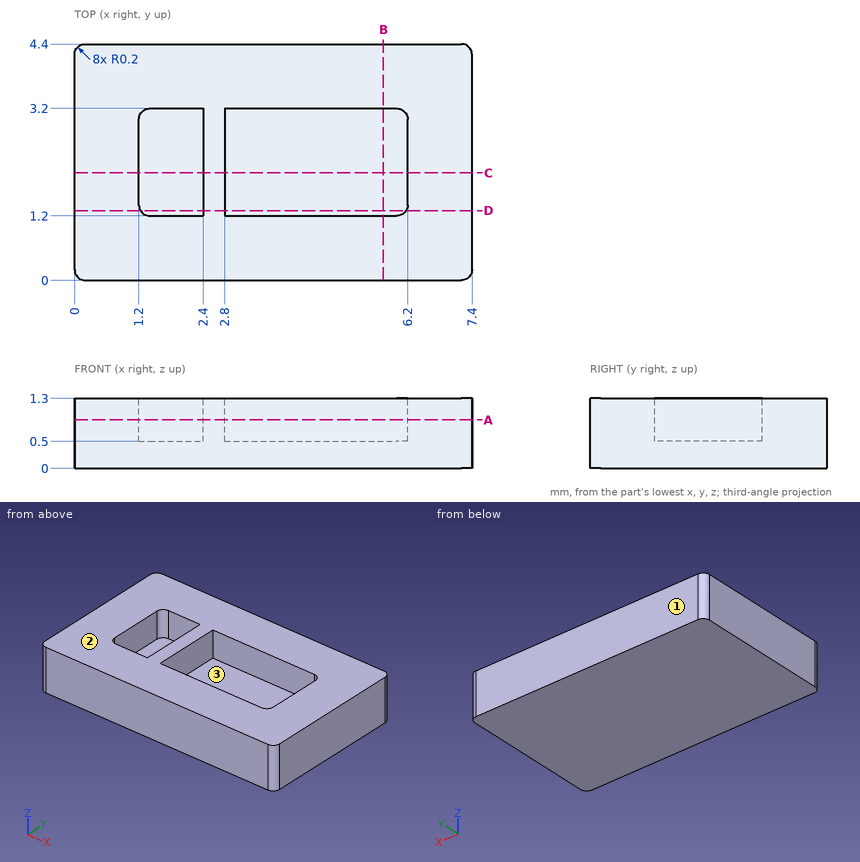
Answer from the drawing. Dimensions are ordinates in mm from the lowest x, y and z of the part. Give positions to 0.01 mm unless a question says otherwise; leave off trailing zeros. Order: outer loops, then holes, each group sorted by start corner. A loop starts at its lowest first (then second) coordinate and runs counter-clockwise, first axis right, second up. Notation, with made-up numbers: (68.5, -21.5) -> (84.5, -21.5) arc R27 ccw to (84.5, 0.5) -> close; hole circle Ø4 at (39, -32.5). An arc over 180 degrees is marked (long way). Answer as a JSON object with one key per item and string values. Group by question number.
1. A flat-ended cylindrical pin translates along its axis: pin 1 Ø0.6 at (y, z) = (2, 1) entering from -X. Find the tip coordinate at first contact, or state that the pin passes through.
2. The mould has two halves that part along Y. Classify the marked faces 1, 2 and 3: released by +Y, released by -Y, zero draft, split by the parting line, or undercut.
3. Section D-D on y = 1.3 is taken. Determine the outline of the cut face in (x, z).
4. Section A-A on z = 0.9 is taken. Determine the outline of the cut face in (x, y), plus the area to 3 significant figures.
5. Section C-C on y = 2 is taken. Determine the outline of the cut face in (x, z), plus the area to 3 significant figures.
6. Consider line 1 along X through (y, z) = (2, 1.15); line 2 along Y through (x, z) = (5.5, 0.6); line 3 along Z through (x, y) = (1.75, 2.55). Determine where each line is inside the solid, lowest interval first. Write a range as [from, to].
7. Section B-B on x = 5.75 is taken. Determine the outline of the cut face in (y, z).
Result sheet:
{
 "1": {"pin 1": "stops at x = 0"},
 "2": {"face 1": "released by +Y", "face 2": "zero draft", "face 3": "undercut"},
 "3": {"outline": "(0, 0) -> (7.4, 0) -> (7.4, 1.3) -> (6.17, 1.3) -> (6.17, 0.5) -> (2.8, 0.5) -> (2.8, 1.3) -> (2.4, 1.3) -> (2.4, 0.5) -> (1.23, 0.5) -> (1.23, 1.3) -> (0, 1.3) -> close"},
 "4": {"outline": "(0, 0.2) arc R0.2 ccw to (0.2, 0) -> (7.2, 0) arc R0.2 ccw to (7.4, 0.2) -> (7.4, 4.2) arc R0.2 ccw to (7.2, 4.4) -> (0.2, 4.4) arc R0.2 ccw to (0, 4.2) -> close; hole (1.2, 1.4) arc R0.2 ccw to (1.4, 1.2) -> (2.4, 1.2) -> (2.4, 3.2) -> (1.4, 3.2) arc R0.2 ccw to (1.2, 3) -> close; hole (2.8, 1.2) -> (6, 1.2) arc R0.2 ccw to (6.2, 1.4) -> (6.2, 3) arc R0.2 ccw to (6, 3.2) -> (2.8, 3.2) -> close", "area": "23.4 mm^2"},
 "5": {"outline": "(0, 0) -> (7.4, 0) -> (7.4, 1.3) -> (6.2, 1.3) -> (6.2, 0.5) -> (2.8, 0.5) -> (2.8, 1.3) -> (2.4, 1.3) -> (2.4, 0.5) -> (1.2, 0.5) -> (1.2, 1.3) -> (0, 1.3) -> close", "area": "5.94 mm^2"},
 "6": {"line 1": "x = [0, 1.2], [2.4, 2.8], [6.2, 7.4]", "line 2": "y = [0, 1.2], [3.2, 4.4]", "line 3": "z = [0, 0.5]"},
 "7": {"outline": "(0, 0) -> (4.4, 0) -> (4.4, 1.3) -> (3.2, 1.3) -> (3.2, 0.5) -> (1.2, 0.5) -> (1.2, 1.3) -> (0, 1.3) -> close"}
}
